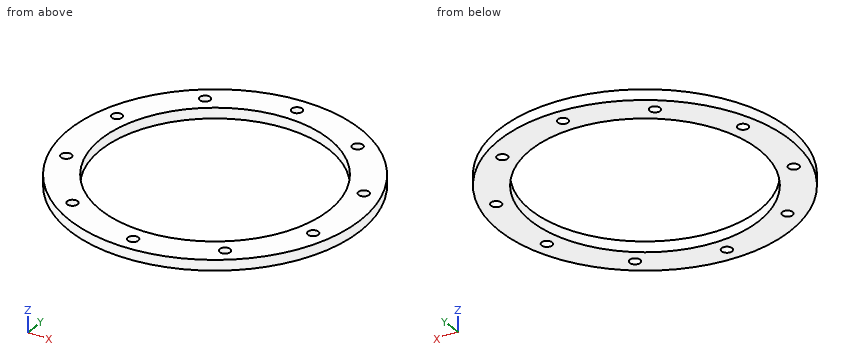
Autodesk Inventor part; units mm, degrees
ref_plane "YZ Plane" through (0, 0, 0) normal (1, 0, 0) x (0, 1, 0)
ref_plane "XZ Plane" through (0, 0, 0) normal (0, 1, 0) x (-1, 0, 0)
ref_plane "XY Plane" through (0, 0, 0) normal (0, 0, 1) x (1, 0, 0)
ref_plane "Work Plane1" through (0, 0, 0) normal (0, 0, 1) x (1, 0, 0)
sketch "Sketch1" plane through (0, 0, 0) normal (0, 0, 1) x (1, 0, 0)
  circle A0 centre (-29.1541, -40.1272) radius 2
  circle A1 centre (-47.1724, -15.3272) radius 2
  circle A2 centre (-47.1724, 15.3272) radius 2
  circle A3 centre (-29.1541, 40.1272) radius 2
  circle A4 centre (0, 49.6) radius 2
  circle A5 centre (29.1541, 40.1272) radius 2
  circle A6 centre (47.1724, 15.3272) radius 2
  circle A7 centre (47.1724, -15.3272) radius 2
  circle A8 centre (29.1541, -40.1272) radius 2
  circle A9 centre (0, -49.6) radius 2
  circle A10 centre (0, 0) radius 55.6
  circle A11 centre (0, 0) radius 43.6
  dimension "d0" = 12
extrude "Extrusion1" add sketch "Sketch1" along normal blind 4
properties part number "Anglerfish_3inch_tube_pressurering"
Input: part model. Units: mm. Frame: model coordinates. Coordinates: 2 decimals unless noted, no trailing zeros. Order: outer loops, then holes, each group sorted by start corner. A loop starts at its lowest first (then second) coordinate and runs counter-clockwise, first axis right, second up. Notation, with made-up numbers: (-31.75, 7) - (4.25, 7) arc R25 cw to (4.25, 34) - close; hole circle Ø1 at (69, 38). An arc over 180 degrees is marked (long way). Put each result on its own line as item: value.
1. Line query: line 1 along Y through (x, z) = (0, 0.8); line 2 along Y through (x, z) = (-47.5, 3.45); line 3 along X through (y, z) = (-40, 0.55). Output: solid intervals per line, ascending.
Report:
line 1: y = -55.6 to -51.6, -47.6 to -43.6, 43.6 to 47.6, 51.6 to 55.6
line 2: y = -28.9 to -17.3, -13.35 to 13.35, 17.3 to 28.9
line 3: x = -38.62 to -31.15, -27.16 to -17.35, 17.35 to 27.16, 31.15 to 38.62
2. Cut plane B-B on x = 0. Return the cut outline in (y, z), then the cut area to 3 significant figures.
Report:
outline: (-55.6, 0) - (-51.6, 0) - (-51.6, 4) - (-55.6, 4) - close; (-47.6, 0) - (-43.6, 0) - (-43.6, 4) - (-47.6, 4) - close; (43.6, 0) - (47.6, 0) - (47.6, 4) - (43.6, 4) - close; (51.6, 0) - (55.6, 0) - (55.6, 4) - (51.6, 4) - close
area: 64.0 mm2
3. Cut plane D-D on z = 0.8. State how many separate pieces and enclosed holes the cut face has, then the cut area to 3 significant figures.
Report:
separate pieces: 1
enclosed holes: 11
area: 3,610 mm2
4. Contact query for flat-ended pins moving along their axis: pin 1 Ø3.5 at (x, y) = (-47.17, -15.33) entering from +Z; pin 2 Ø2 at (x, z) = (26, 1) entering from +Y; pin 3 Ø2 at (y, z) = (3, 3) entering from +X; pin 4 Ø2 at (y, z) = (-21.5, 2.5) entering from -X. Output: stop coordinate, or through.
Report:
pin 1: passes through
pin 2: stops at y = 49.66
pin 3: stops at x = 55.56
pin 4: stops at x = -51.68
5. Cut plane A-A on y = 0. Return the cut outline in (x, z).
Report:
outline: (-55.6, 0) - (-43.6, 0) - (-43.6, 4) - (-55.6, 4) - close; (43.6, 0) - (55.6, 0) - (55.6, 4) - (43.6, 4) - close
6. Cut plane C-C on x = -17. Return the cut outline in (y, z).
Report:
outline: (-52.94, 0) - (-40.15, 0) - (-40.15, 4) - (-52.94, 4) - close; (40.15, 0) - (52.94, 0) - (52.94, 4) - (40.15, 4) - close
